```python
from build123d import *

# Parameters (mm, degrees)
F0_R     = 50
F1_DEPTH = 50
F2_R     = 45
F3_DEPTH = 80
F5_DEPTH = 100
F6_R     = 17.5
F7_DEPTH = 100


with BuildPart() as f1:
    # F0 (on Front) → F1 (new body)
    with BuildSketch(Plane.XZ):
        Circle(F0_R)
    extrude(amount=-F1_DEPTH)

    # F2 (on face) → F3 (join)
    with BuildSketch(Plane(origin=(0, 50, 0), x_dir=(-1, 0, 0), z_dir=(0, 1, 0))):
        Circle(F2_R)
    extrude(amount=F3_DEPTH)

    # F4 (on Top) → F5 (cut, symmetric)
    with BuildSketch(Plane.XY):
        with BuildLine():
            ThreePointArc((-35, 90), (0, 55), (35, 90))
            ThreePointArc((35, 90), (0, 125), (-35, 90))
        make_face()
        with BuildLine():
            ThreePointArc((-35, 90), (0, 125), (35, 90))
            Line((35, 90), (35, 130))
            Line((35, 130), (-35, 130))
            Line((-35, 130), (-35, 90))
        make_face()
    extrude(amount=F5_DEPTH, both=True, mode=Mode.SUBTRACT)

    # F6 (on face) → F7 (cut, symmetric)
    with BuildSketch(Plane.YZ.offset(-35)):
        with Locations((90, 0)):
            Circle(F6_R)
        with BuildLine():
            ThreePointArc((90, 28.2842712475), (118.2842712475, 0), (90, -28.2842712475))
            Line((90, -28.2842712475), (130, -28.2842712475))
            Line((130, -28.2842712475), (130, 28.2842712475))
            Line((130, 28.2842712475), (90, 28.2842712475))
        make_face()
    extrude(amount=F7_DEPTH, both=True, mode=Mode.SUBTRACT)


solid = f1.part
```
Work out the finished part from the listing and answer in its coordinate system (mm). A direction names the side the tool comes from. Give positions to 0.01 mm unless a question says otherwise; leave off trailing zeros. Loops run counter-clockwise (first coordinate to the right, second up) from the corner with the lowest first, then second, coordinate; pieces in that order, holes last. Notation, with made-up numbers: (75.5, 52.5) - (84.5, 52.5) arc R27 ccw to (84.5, 90.5) - close; hole circle Ø3 at (-6, 46). An arc over 180 degrees is marked (long way). Use CSV: the item, a comma, the result in double quotes. Start each with the question number.
(1) Find section A-A, the plane z = 0. Determine the outline of the cut face in (x, y).
(2) A tool of negligible diameter and unlimited length cuts with its end or side. For faces 4 (the face through (-41, 50, 19)), 5 (the face through (-35, 111, 0)), 6 (the face through (-38.819, 118.277, 0.622)), from which of +Z, -Z, +X, -X, +Y, -Y can it reach the whole face along a straight path? Write none if from no direction.
(3) Find the intervals of material crossed by L1, parallel to Y at x = 42, z = 0; L2, parallel to Z at x = 38.25, y = 90; L3, parallel to Y at x = -45.5, z = 1.5, in increasing order.
(4) Each of these flat-tipped pins is pushed along its axis until it touches: pin 1 (8.5 mm diameter, centred on y = 106, z = 3, fed in from +X); pin 2 (5 mm diameter, centred on x = -21.5, y = 33.5, fed in from -Z); pin 3 (6 mm diameter, centred on x = 31.5, y = 61.5, fed in from -Z). Where does it stop, or does it pass through?
(5) Determine the mould class of faces 1 (the face through (38.959, 118.277, 0.622)), 2 (the face through (47.69, 24.65, 15.02)), 3 (the face through (-39.185, 72.517, 0.769)) for opening direction Y: released by +Y, released by -Y, zero draft, split by the parting line, or undercut.
(6) Find section C-C, the plane x = 0. Determine the outline of the cut face in (y, z), plus the area to 3 significant figures.
(7) Find section B-B, the plane y = 88.5. Determine the outline of the cut face in (x, z).
(8) Find section D-D, the plane x = 38.5. Determine the outline of the cut face in (y, z), plus the area to 3 significant figures.
Results found:
1,outline,"(-50, 0) - (50, 0) - (50, 50) - (45, 50) - (45, 72.5) - (30.31, 72.5) arc R35 cw to (-30.31, 72.5) - (-45, 72.5) - (-45, 50) - (-50, 50) - close; (-45, 107.5) - (-35, 107.5) - (-35, 118.28) - (-45, 118.28) - close; (35, 107.5) - (45, 107.5) - (45, 118.28) - (35, 118.28) - close"
2,face 4,"+Y"
2,face 5,"+Z, -Z, +Y"
2,face 6,"+X, -X, +Y"
3,L1,"0 to 72.5, 107.5 to 118.28"
3,L2,"-23.71 to -17.5, 17.5 to 23.71"
3,L3,"0 to 50"
4,pin 1,"x = 45"
4,pin 2,"z = -46.25"
4,pin 3,"z = -34.82"
5,face 1,"released by +Y"
5,face 2,"zero draft"
5,face 3,"undercut"
6,outline,"(0, -50) - (50, -50) - (50, -45) - (55, -45) - (55, 45) - (50, 45) - (50, 50) - (0, 50) - close"
6,area,"5,450 mm^2"
7,outline,"(-41.48, -17.44) arc R45 ccw to (-34.97, -28.32) - (-34.97, -17.44) - close; (-41.48, 17.44) - (-34.97, 17.44) - (-34.97, 28.32) arc R45 ccw to start; (34.97, -28.32) arc R45 ccw to (41.48, -17.44) - (34.97, -17.44) - close; (34.97, 17.44) - (41.48, 17.44) arc R45 ccw to (34.97, 28.32) - close"
8,outline,"(0, -31.9) - (50, -31.9) - (50, -23.3) - (106.04, -23.3) arc R28.28 ccw to (106.04, 23.3) - (50, 23.3) - (50, 31.9) - (0, 31.9) - close; hole circle Ø35 at (90, 0)"
8,area,"5,240 mm^2"
